Part model, mm, in its own coordinate system. A direction names the side the tool comes from. Give positions to 0.01 mm unless a question says otherwise; leave off trailing zeros. Loops run counter-clockwise (first coordinate to the right, second up) from the corner with the lowest first, then second, coordinate; pieces in that order, holes last. Notation, with made-up numbers: (82, 39.5) -> (119, 39.5) arc R25 cw to (119, 78.5) -> close; hole circle Ø2 at (54, 34.25). An arc over 180 degrees is marked (long way). Write item = value, one per line.
from build123d import *

# Parameters (mm, degrees)
SKETCH002_R  = 30
PAD004_DEPTH = 9
THICKNESS_T  = -1
CHAMFER_SIZE = 0.5
POCKET_DEPTH = 30.001


with BuildPart() as part:
    # Sketch002 → Pad004 (new body)
    with BuildSketch(Plane.XY):
        Circle(SKETCH002_R)
    extrude(amount=PAD004_DEPTH)

    # Thickness
    thickness_openings = [part.faces().sort_by_distance(p)[0] for p in [
        (0, 0, 0),
    ]]
    offset(amount=THICKNESS_T, openings=thickness_openings)

    # Chamfer
    chamfer_edges = [part.edges().sort_by_distance(p)[0] for p in [
        (-30, 0, 9),
    ]]
    chamfer(chamfer_edges, length=CHAMFER_SIZE)

    # Sketch003 → Pocket (cut, through all)
    with BuildSketch(Plane.YZ):
        with BuildLine():
            ThreePointArc((2.291288, 0), (0, 3.5), (-2.291288, 0))
            Line((-2.291288, 0), (2.291288, 0))
        make_face()
    extrude(amount=-POCKET_DEPTH, mode=Mode.SUBTRACT)


solid = part.part
1) Slice it at A-A, the plane y = 0. List the corners of the cut face in (x, z), and give its area (4 significant figures).
Resolved:
outline = (-30, 3.5) -> (-29, 3.5) -> (-29, 8) -> (29, 8) -> (29, 0) -> (30, 0) -> (30, 8.5) -> (29.5, 9) -> (-29.5, 9) -> (-30, 8.5) -> close
area = 72.25 mm²
2) Slice it at D-D, the plane z = 2.25. List the corners of the cut face in (x, y), and give its area (3 significant figures).
Resolved:
outline = (-29.92, -2.17) arc R30 ccw (long way) to (-29.92, 2.17) -> (-28.92, 2.17) arc R29 cw (long way) to (-28.92, -2.17) -> close
area = 181 mm²
3) Drop flat-ended pins along their axis: P1, Ø4, axis at x = -15, y = -17.5, coming from the -Z side; P2, Ø2, axis at y = 2, z = 2, coming from the +X side; P3, Ø1, axis at x = 18.5, z = 2, coming from the +Y side. Give the stop position or say it passes through.
Resolved:
P1 = 8
P2 = 29.98
P3 = 24
4) Slice it at B-B, the plane x = 0. List the corners of the cut face in (y, z).
Resolved:
outline = (-30, 0) -> (-29, 0) -> (-29, 8) -> (29, 8) -> (29, 0) -> (30, 0) -> (30, 8.5) -> (29.5, 9) -> (-29.5, 9) -> (-30, 8.5) -> close
5) Drill centre lines: line 1 along X through (y, z) = (0, 6.25); line 2 along Z through (x, y) = (-12, -5); line 3 along X through (y, z) = (0, 2). Where is each one in solid material? Low to high. Write a range as [from, to].
Resolved:
line_1 = [-30, -29], [29, 30]
line_2 = [8, 9]
line_3 = [29, 30]
6) Slice it at C-C, the plane z = 5.25. List the corners of the cut face in (x, y).
Resolved:
outline = circle Ø60 at (0, 0); hole circle Ø58 at (0, 0)
7) Pull direction Y, two halves, no side cores. Call faces 1 (the face through (27.712, -11.49, 4.19)), 2 (the face through (-29.4, 0.1, 3.5)), 3 (the face through (-11, 27, 0)), 4 (the face through (0, 0, 8)): pulls with the +Y half, pulls with the -Y half, needs draft (parallel to the pull), parting line crosses it, or undercut.
Resolved:
face_1 = parting line crosses it
face_2 = undercut
face_3 = needs draft
face_4 = undercut
8) Which spindle directions (+Z, -Z, +X, -X, +Y, -Y) get a long thin tool onto all of the face, cutting with end or side? Do faces 5 (the face through (0, 0, 9)), 6 (the face through (26.789, -11.107, 3.944)). Say none if no direction does.
Resolved:
face_5 = +Z, +X, -X, +Y, -Y
face_6 = -Z
